Input: part model. Units: mm. Frame: model coordinates. A direction names the side the tool comes from. Give positions to 0.01 mm unless a question says otherwise; leave off trailing zeros. Order: outer loops, then holes, each group sorted by start corner. A loop starts at its lowest first (then second) coordinate and runs counter-clockwise, first axis right, second up. Notation, with made-up numbers: (2.5, 20.25) - (30.5, 20.25) arc R12 cw to (30.5, 40.25) - close; hole circle Ø1 at (0.5, -36). An arc over 180 degrees is marked (long way). Answer in a Markdown table with one row per item. Add a question column.
from build123d import *

# Parameters (mm, degrees)
F0_W          = 1800
F0_H          = 1060
F1_DEPTH      = 12
F3_W          = 333.5
F3_H          = 12
F4_DEPTH      = 176
F6_DEPTH      = 176
F8_DEPTH      = 566.5
F8_DEPTH_BACK = 566.5
F9_W          = 1133
F9_H          = 686
F10_DEPTH     = 25
F11_W         = 1133
F11_H         = 12
F12_DEPTH     = 176
F13_W         = 321.5
F13_H         = 1036
F14_DEPTH     = 12
F15_W         = 1133
F15_H         = 12
F16_DEPTH     = 343
F17_DEPTH     = 343
F18_W         = 1133
F18_H         = 12
F19_DEPTH     = 65
F21_W         = 164
F21_H         = 12
F22_DEPTH     = 321.5
F23_W         = 164
F23_H         = 12
F24_DEPTH     = 321.5
F25_W         = 1133
F25_H         = 12
F26_DEPTH     = 175
F27_W         = 12
F27_H         = 1060
F28_DEPTH     = 28.5
F29_W         = 12
F29_H         = 1060
F30_DEPTH     = 28.5
F31_DEPTH     = 16.5
F32_DEPTH     = 16.5


with BuildPart() as f1:
    # F0 (on Front) → F1 (new body)
    with BuildSketch(Plane.XZ):
        Rectangle(F0_W, F0_H)
    extrude(amount=F1_DEPTH)

    # F3 (on offset) → F4 (join, through all)
    with BuildSketch(Plane.XZ.offset(-176)):
        with Locations((-733.25, 524)):
            Rectangle(F3_W, F3_H)
        with Locations((733.25, 524)):
            Rectangle(F3_W, F3_H)
    extrude(amount=F4_DEPTH)

    # F5 (on offset) → F6 (join, through all)
    with BuildSketch(Plane.XZ.offset(-176)):
        Polygon((578.5, -518), (578.5, 518), (566.5, 518), (566.5, -530), (900, -530), (900, -518), align=None)
        Polygon((-900, -518), (-900, -530), (-566.5, -530), (-566.5, 518), (-578.5, 518), (-578.5, -518), align=None)
    extrude(amount=F6_DEPTH)

    # F7 (on Right) → F8 (join, two sides)
    with BuildSketch(Plane.YZ) as f8_sk:
        Polygon((176, 273), (176, 343), (96, 343), (96, 303), (136, 303), (136, 273), align=None)
    extrude(amount=F8_DEPTH)
    extrude(f8_sk.sketch, amount=-F8_DEPTH_BACK)

    # F9 (on face) → F10 (cut)
    with BuildSketch(Plane.XZ.offset(12)):
        Rectangle(F9_W, F9_H)
    extrude(amount=-F10_DEPTH, mode=Mode.SUBTRACT)

    # F11 (on face) → F12 (join, through all)
    with BuildSketch(Plane.XZ):
        with Locations((0, 349)):
            Rectangle(F11_W, F11_H)
    extrude(amount=-F12_DEPTH)

    # F13 (on face) → F14 (join)
    with BuildSketch(Plane(origin=(0, 176, 0), x_dir=(-1, 0, 0), z_dir=(0, 1, 0))):
        with Locations((739.25, 0)):
            Rectangle(F13_W, F13_H)
        with Locations((-739.25, 0)):
            Rectangle(F13_W, F13_H)
    extrude(amount=-F14_DEPTH)

    # F15 (on Top) → F16 (join, through all)
    with BuildSketch(Plane.XY):
        with Locations((0, 59)):
            Rectangle(F15_W, F15_H)
    extrude(amount=F16_DEPTH)

    # F15 (on Top) → F17 (join, through all)
    with BuildSketch(Plane.XY):
        with Locations((0, 59)):
            Rectangle(F15_W, F15_H)
    extrude(amount=-F17_DEPTH)

    # F18 (on face) → F19 (join, through all)
    with BuildSketch(Plane(origin=(0, 0, 0), x_dir=(-1, 0, 0), z_dir=(0, 1, 0))):
        with Locations((0, -349)):
            Rectangle(F18_W, F18_H)
    extrude(amount=F19_DEPTH)

    # F21 (on face) → F22 (join, through all)
    with BuildSketch(Plane(origin=(-578.5, 0, 0), x_dir=(0, -1, 0), z_dir=(-1, 0, 0))):
        with Locations((-82, -112)):
            Rectangle(F21_W, F21_H)
        with Locations((-82, 200)):
            Rectangle(F21_W, F21_H)
    extrude(amount=F22_DEPTH)

    # F23 (on face) → F24 (join, through all)
    with BuildSketch(Plane.YZ.offset(578.5)):
        with Locations((82, -112)):
            Rectangle(F23_W, F23_H)
        with Locations((82, 200)):
            Rectangle(F23_W, F23_H)
    extrude(amount=F24_DEPTH)

    # F25 (on face) → F26 (join, through all)
    with BuildSketch(Plane.XY.offset(355)):
        with Locations((0, 170)):
            Rectangle(F25_W, F25_H)
    extrude(amount=F26_DEPTH)

    # F27 (on face) → F28 (join)
    with BuildSketch(Plane(origin=(-900, 0, 0), x_dir=(0, -1, 0), z_dir=(-1, 0, 0))):
        with Locations((6, 0)):
            Rectangle(F27_W, F27_H)
    extrude(amount=F28_DEPTH)

    # F29 (on face) → F30 (join)
    with BuildSketch(Plane.YZ.offset(900)):
        with Locations((-6, 0)):
            Rectangle(F29_W, F29_H)
    extrude(amount=F30_DEPTH)

    # F31 (add): a face of the model
    f31_faces = [f1.faces().sort_by_distance(p)[0] for p in [
        (900, 88, -519.2548801775),
    ]]
    extrude(f31_faces, amount=F31_DEPTH)

    # F32 (add): a face of the model
    f32_faces = [f1.faces().sort_by_distance(p)[0] for p in [
        (-900, 88, 519.2548801775),
    ]]
    extrude(f32_faces, amount=F32_DEPTH)


solid = f1.part
Q1. Section B-B, the plane x = 804. Return loops of the section in (y, z), then the cut area to 3 significant figures.
Q2. Pull-direction query (X, two-part tool) for faces 1 (the flat face through (-578.5, 83, -315)), 2 (the flat face through (13, 176, 361)), 3 (the flat face through (-566.5, 109, -197)), 4 (the flat face through (8, 116, 303)); classes: +X half, -X half, draft (parallel to the pull), parting line (faces both ways), or undercut.
Q3. Section C-C, the plane z = 322. Return loops of the section in (x, y), then the cut area to 3 significant figures.
Q4. Section A-A, the plane z = -281.5. Return loops of the section in (x, y).
Q5. Section D-D, the plane x = 424.5. Return loops of the section in (y, z).
Q6. Access query for faces 5 (the flat face through (745, 164, 42)), 6 (the flat face through (-8, 0, 444)), 7 (the flat face through (-745, 83, -106)). Directions: +Z, -Z, +X, -X, +Y, -Y. A direction counts if a zero-diameter tool reaches every point of the face in a straight line with its end or side. Return the directions, or none.
Q7. Contact query for flat-ended pins moving along their axis: P1, Ø5, axis at x = 293, z = 237, coming from the +Y side; P2, Ø6, axis at x = -233.5, z = 219, coming from the -Y side; P3, Ø10, axis at y = 115.5, z = 139, coming from the +X side. Output: stop coordinate, or through.
Q8. Line query: probe 1 along Z at (x, y) = (-634, 6.5); probe 2 along Y at (x, z) = (344, 289.5); probe 3 along X at (y, z) = (83, -99.5). Output: solid intervals per line, ascending.
Computed:
| question | item | result |
|---|---|---|
| 1 | outline | (-12, -530) - (176, -530) - (176, 530) - (-12, 530) - close; hole (0, -518) - (164, -518) - (164, -118) - (0, -118) - close; hole (0, -106) - (164, -106) - (164, 194) - (0, 194) - close; hole (0, 206) - (164, 206) - (164, 518) - (0, 518) - close |
| 1 | area | 33,300 mm^2 |
| 2 | face 1 | -X half |
| 2 | face 2 | draft |
| 2 | face 3 | undercut |
| 2 | face 4 | undercut |
| 3 | outline | (-928.5, -12) - (-566.5, -12) - (-566.5, 53) - (566.5, 53) - (566.5, -12) - (928.5, -12) - (928.5, 0) - (578.5, 0) - (578.5, 164) - (916.5, 164) - (916.5, 176) - (-916.5, 176) - (-916.5, 164) - (-578.5, 164) - (-578.5, 0) - (-928.5, 0) - close; hole (-566.5, 65) - (566.5, 65) - (566.5, 96) - (-566.5, 96) - close |
| 3 | area | 125,000 mm^2 |
| 4 | outline | (-928.5, -12) - (-566.5, -12) - (-566.5, 53) - (566.5, 53) - (566.5, -12) - (928.5, -12) - (928.5, 0) - (578.5, 0) - (578.5, 164) - (916.5, 164) - (916.5, 176) - (566.5, 176) - (566.5, 65) - (-566.5, 65) - (-566.5, 176) - (-916.5, 176) - (-916.5, 164) - (-578.5, 164) - (-578.5, 0) - (-928.5, 0) - close |
| 5 | outline | (-12, -530) - (0, -530) - (0, -355) - (65, -355) - (65, 343) - (96, 343) - (96, 303) - (136, 303) - (136, 273) - (176, 273) - (176, 530) - (164, 530) - (164, 355) - (0, 355) - (0, 530) - (-12, 530) - (-12, 343) - (53, 343) - (53, -343) - (-12, -343) - close |
| 6 | face 5 | +X |
| 6 | face 6 | +Z |
| 6 | face 7 | -X |
| 7 | P1 | stops at y = 65 |
| 7 | P2 | stops at y = 53 |
| 7 | P3 | stops at x = 578.5 |
| 8 | probe 1 | z = -530 to -518, -118 to -106, 194 to 206, 518 to 530 |
| 8 | probe 2 | y = 53 to 65, 136 to 176 |
| 8 | probe 3 | x = -578.5 to -566.5, 566.5 to 578.5 |
